Could you check a few things on this model? Use its own coordinates, in mm. Coordinates: 2 decimals unless noted, no trailing zeros. Loops run counter-clockwise (first coordinate to the right, second up) from the corner with the lowest first, then second, coordinate; pieces in that order, holes last. Notation, with made-up numbers: M 85,71.25 L 93,71.25 A18 cw 93,106.25 Z; hole C 38.5,30 d5. An arc over 180 degrees is marked long. Write each question's results on one line, items separated by ' | '.
```python
from build123d import *

# Parameters (mm, degrees)
ESQUISSE1_W             = 70
ESQUISSE1_H             = 30
BOSS_EXTRU_1_DEPTH      = 20
CONG_7_R                = 10
ESQUISSE12_R            = 1.25
ENL_V_MAT_EXTRU_5_DEPTH = 15
ESQUISSE11_R            = 1.25
ENL_V_MAT_EXTRU_6_DEPTH = 20


with BuildPart() as part:
    # Esquisse1 → Boss.-Extru.1 (new body, symmetric)
    with BuildSketch(Plane.XY):
        with BuildLine():
            ThreePointArc((79.782402832, -100), (75.641274878, -35.393198769), (35, 15))
            Line((35, 15), (35, -15))
            Line((35, -15), (-35, -15))
            ThreePointArc((-35, -15), (36.414284285, -38.56349239), (79.782402832, -100))
        make_face()
        Rectangle(ESQUISSE1_W, ESQUISSE1_H)
    extrude(amount=BOSS_EXTRU_1_DEPTH, both=True)

    # Congé7
    cong_7_edges = [part.edges().sort_by_distance(p)[0] for p in [
        (-35, 0, 20),
        (75.641274878, -35.393198769, 20),
        (-35, 0, -20),
        (0, 15, -20),
        (75.641274878, -35.393198769, -20),
        (0, 15, 20),
        (-35, 15, 0),
        (35, 15, 0),
    ]]
    fillet(cong_7_edges, radius=CONG_7_R)

    # Esquisse12 → Enlèv. mat.-Extru.5 (cut)
    with BuildSketch(Plane(origin=(0, -18.687162838, 0), x_dir=(1, 0, 0), z_dir=(0, 1, 0))):
        with Locations((-21.600806316, 0)):
            Circle(ESQUISSE12_R)
    extrude(amount=ENL_V_MAT_EXTRU_5_DEPTH, mode=Mode.SUBTRACT)

    # Esquisse11 → Enlèv. mat.-Extru.6 (cut)
    with BuildSketch(Plane(origin=(0, -54.41956978, 0), x_dir=(1, 0, 0), z_dir=(0, 1, 0))):
        with Locations((47.550679202, 0)):
            Circle(ESQUISSE11_R)
    extrude(amount=ENL_V_MAT_EXTRU_6_DEPTH, mode=Mode.SUBTRACT)


solid = part.part
```
(1) Imagine slicing it at B-B, the plane x = 1. List the corners of the cut face in (y, z) for me, and give its area (3 significant figures).
Reported:
outline: M -20.53,-20 L 5,-20 A10 ccw 15,-10 L 15,10 A10 ccw 5,20 L -20.53,20 Z | area: 1,380 mm2
(2) Imagine slicing it at A-A, the plane z = 14.5. List the corners of the cut face in (x, y) for me, and give its area (3 significant figures).
Reported:
outline: M -33.93,-15 A120 cw 79.16,-98.01 A105.93 ccw 37.06,12.29 A8.93 ccw 31.91,13.93 L -25,13.93 A8.93 ccw -33.93,5 Z | area: 4,840 mm2
(3) Please list where these lines run through material, in increasing order: probe 1 along X at (y, z) = (-41.25, 0); probe 2 along X at (y, z) = (-45, 0); probe 3 along Z at (x, y) = (43.5, 0). Write a range as from..to.
Reported:
probe 1: x = 39.91..46.3, 48.8..77.73 | probe 2: x = 44.37..46.3, 48.8..78.87 | probe 3: z = -19.42..19.42
(4) Will these pins go through, and if not, where does the flat tip stop? P1, Ø12, axis at x = 61.5, z = 10.5, coming from the +Y side; P2, Ø4, axis at x = 47, z = 1.5, coming from the +Y side; P3, Ø12, axis at y = -24, z = -4.5, coming from the +X side.
Reported:
P1: stops at y = -2.69 | P2: stops at y = 7.5 | P3: stops at x = 73.37
